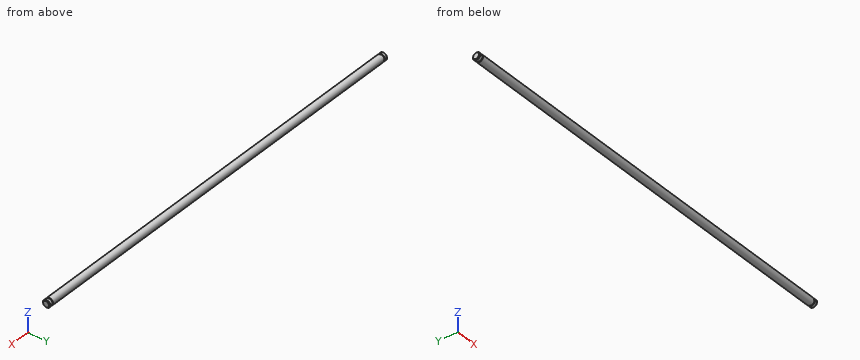
from build123d import *

# Parameters (mm, degrees)
CHAMFER1_SIZE = 0.508


with BuildPart() as part:
    # Sketch1 → Revolve1 (revolve)
    with BuildSketch(Plane.XY):
        Polygon((-152.7556, 0), (116.3066, 0), (116.3066, 2.38125), (114.2746, 2.38125), (114.2746, 1.8669), (113.538, 1.8669), (113.538, 2.38125), (-149.987, 2.38125), (-149.987, 1.8669), (-150.7236, 1.8669), (-150.7236, 2.38125), (-152.7556, 2.38125), align=None)
    revolve(axis=Axis((116.3066, 0, 0), (1, 0, 0)))

    # Chamfer1
    chamfer1_edges = [part.edges().sort_by_distance(p)[0] for p in [
        (-152.7556, -2.38125, 0),
        (116.3066, -2.38125, 0),
    ]]
    chamfer(chamfer1_edges, length=CHAMFER1_SIZE)


solid = part.part
Geometry check sheet. Reference: the model listing, model coordinates, mm. Coordinates: 2 decimals unless noted, no trailing zeros. Order: outer loops, then holes, each group sorted by start corner. A loop starts at its lowest first (then second) coordinate and runs counter-clockwise, first axis right, second up. Notation, with made-up numbers: (9.25, -4) - (23.25, -4) arc R21 ccw to (23.25, 17) - close; hole circle Ø3 at (41.5, 36). An arc over 180 degrees is marked (long way). Answer in a Markdown table with one row per item. Add a question column.
1) Material ranges on line 1 along X through (y, z) = (-2, -0.6); line 2 along Z through (x, y) = (-62.5, 0.2); line 3 along Y through (x, z) = (-82.5, 0.4), recorded low to high. Write a range as [from, to].
2) Cross-section at A-A, the plane x = -82.5. Record the cut outline in (y, z), then the cut area to 3 significant figures.
3) Gauge pin test, flat end, axial feed: P1, Ø1.5, axis at x = -13.5, z = 1, coming from the +Y side. Record the tip position at first contact, or that the pin passes through.
Check result:
| question | item | result |
|---|---|---|
| 1 | line 1 | x = [-152.54, -150.72], [-149.99, 113.54], [114.27, 116.09] |
| 1 | line 2 | z = [-2.37, 2.37] |
| 1 | line 3 | y = [-2.35, 2.35] |
| 2 | outline | circle Ø4.76 at (0, 0) |
| 2 | area | 17.8 mm² |
| 3 | P1 | stops at y = 2.37 |
